Source: CAD feature listing. Evaluate the final solid. Frame: model axes, mm. Face numbers are marked on the shaded views. A direction names the side the tool comes from. Round coordinates to 2 decimals unless told otherwise and drop trailing zeros. Write each loop counter-clockwise with the first axis right and the second up, starting at its lowest first coordinate (ties: lowest second). Pieces come first, ordered by that corner, then holes. Notation, with made-up numbers: M 16.25,60 L 38.25,60 A19 cw 38.25,92 Z; hole C -36,81.25 d3. An arc over 180 degrees is marked long. Put each result on its own line as item: value. Start each with the question number.
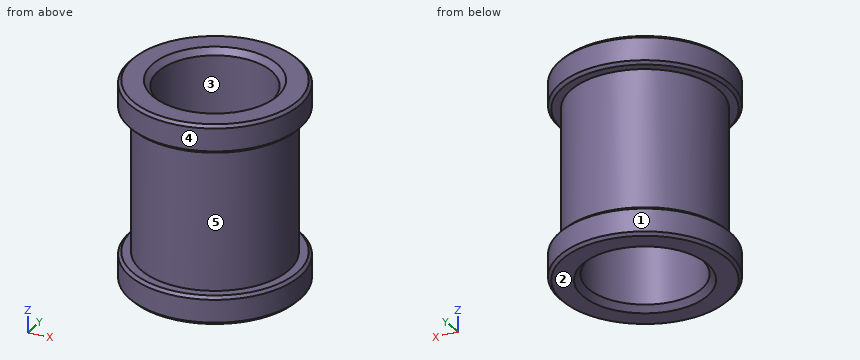
Autodesk Inventor part; units mm, degrees
ref_plane "YZ Plane" through (0, 0, 0) normal (1, 0, 0) x (0, 1, 0)
ref_plane "XZ Plane" through (0, 0, 0) normal (0, 1, 0) x (-1, 0, 0)
ref_plane "XY Plane" through (0, 0, 0) normal (0, 0, 1) x (1, 0, 0)
sketch "Sketch1" plane through (0, 0, 0) normal (0, 0, 1) x (1, 0, 0)
  circle A0 centre (27.2718, 25.897) radius 13
  circle A1 centre (27.2718, 25.897) radius 10
  point P0 (0, 0)
  dimension "d0" = 20
extrude "Extrusion1" add sketch "Sketch1" against normal blind 12.5
sketch "Sketch2" plane through (27.2718, 25.897, 0) normal (0, 0, 1) x (1, 0, 0)
  circle A0 centre (0, 0) radius 15
  circle A1 centre (0, 0) radius 10
  point P0 (-27.2718, -25.897)
  dimension "d4" = 30
extrude "Extrusion2" add sketch "Sketch2" along normal blind 5
mirror "Mirror1" about plane through (27.2718, 25.897, -12.5) normal (0, 0, -1) of "Extrusion1", "Extrusion2"
chamfer "Chamfer1" distance 0.5 angle 45 4 edges at (12.2718, 25.897, -30) (12.2718, 25.897, 5) (12.2718, 25.897, 0) (12.2718, 25.897, -25)
chamfer "Chamfer2" distance 1 angle 45 2 edges at (17.2718, 25.897, 5) (17.2718, 25.897, -30)
properties part number "Holkki" material "Polyethylene, High Density"
(1) Section query A-A (z = -15). Return loops of the section in (x, y), and give its area (3 significant figures).
(2) Contact query for flat-ended pins moving along their axis: P1, Ø2, axis at y = 24, z = -13, coming from the +X side; P2, Ø14.5, axis at x = 22, y = 20.5, coming from the +Z side; P3, Ø1.5, axis at x = 18.5, z = -1.5, coming from the -Y side; P4, Ø4, axis at x = 29.5, z = -10.5, coming from the +Y side (3 decimals). Output: stop coordinate, or through.
(3) Section query B-B (z = -28). Return loops of the section in (x, y), and give its area (3 significant figures).
(4) Ray query, line 1 along Z through (x, y) = (32, 39); line 2 along X through (y, z) = (18, 2.5); line 3 along X through (y, z) = (18.25, -10). Return the intervals inside material, ascending.
(5) Pull-direction query (Y, two-part tool) for the marked faces 1, 2 and 3; classes: +Y half, -Y half, draft (parallel to the pull), parting line (faces both ways), or undercut.
(6) Access query for the marked faces 4 and 5. Directions: +Z, -Z, +X, -X, +Y, -Y. A direction counts if a zero-diameter tool reaches every point of the face in a straight line with its end or side. Return the directions, or none.
Entries:
1. outline: C 27.27,25.9 d26; hole C 27.27,25.9 d20
1. area: 217 mm2
2. P1: x = 40.24
2. P2: z = 5
2. P3: y = 15.67
2. P4: y = 38.895
3. outline: C 27.27,25.9 d30; hole C 27.27,25.9 d20
3. area: 393 mm2
4. line 1: -30 to -25, 0 to 5
4. line 2: 14.52 to 21.14, 33.41 to 40.02
4. line 3: 16.76 to 20.83, 33.72 to 37.78
5. face 1: parting line
5. face 2: draft
5. face 3: undercut
6. face 4: +Z, -Z
6. face 5: none
